Could you check a few things on this model? Use its own coordinates, in mm. A direction names the side the tool comes from. Round coordinates to 2 decimals unless told otherwise and drop trailing zeros. Order: outer loops, then holes, each group sorted by start corner. A loop starts at its lowest first (then second) coordinate and runs counter-clockwise, first axis right, second up. Notation, with made-up numbers: (84.25, 75.5) -> (90.25, 75.5) arc R23 cw to (90.25, 98.5) -> close; hole circle Ø4 at (-38.75, -6.5). An arc over 180 degrees is marked (long way). Put each result on its own line as item: value. Start each with the question number.
from build123d import *

# Parameters (mm, degrees)
BOSS_EXTRUDE1_DEPTH = 50
BOSS_EXTRUDE2_DEPTH = 30


with BuildPart() as part:
    # Sketch1 → Boss-Extrude1 (new body)
    with BuildSketch(Plane(origin=(0, 0, 0), x_dir=(1, 0, 0), z_dir=(0, 1, 0))):
        with BuildLine():
            Line((-1.5875, -2.749630657), (-1.5875, -22.749630657))
            Line((-1.5875, -22.749630657), (-5.5875, -22.749630657))
            Line((-5.5875, -22.749630657), (-5.5875, -4.501163044))
            ThreePointArc((-5.5875, -4.501163044), (0, 7.175), (5.5875, -4.501163044))
            Line((5.5875, -4.501163044), (5.5875, -22.749630657))
            Line((5.5875, -22.749630657), (1.5875, -22.749630657))
            Line((1.5875, -22.749630657), (1.5875, -2.749630657))
            ThreePointArc((1.5875, -2.749630657), (3.175, 0), (1.5875, 2.749630657))
            Line((1.5875, 2.749630657), (-1.5875, 2.749630657))
            ThreePointArc((-1.5875, 2.749630657), (-3.175, 0), (-1.5875, -2.749630657))
        make_face()
    extrude(amount=BOSS_EXTRUDE1_DEPTH)

    # Sketch5 → Boss-Extrude2 (add)
    with BuildSketch(Plane(origin=(0, 50, 0), x_dir=(1, 0, 0), z_dir=(0, 1, 0))):
        Polygon((-5.5875, -22.749630657), (-35.5875, -22.749630657), (-35.5875, -102.749630657), (-1.5875, -102.749630657), (-1.5875, -107.749630657), (-40.5875, -107.749630657), (-40.5875, -16.749630657), (-5.5875, -16.749630657), align=None)
    extrude(amount=-BOSS_EXTRUDE2_DEPTH)


solid = part.part
1. Thinking about a two-plate mould opening in X: for faces 5 (the face through (-1.588, 25, 13)), 6 (the face through (-40.588, 35, 63)), 7 (the face through (-36, 50, 50)), which applies, +X half, -X half, draft (parallel to the pull), parting line (faces both ways), or undercut?
2. If we section it at D-D, the plane z = 99: Please give me the cut outline in (x, y).
3. If we section it at B-B, the plane z = 12: Please give me the cut outline in (x, y).
4. For pin 1 Ø8 at (y, z) = (13, 12) entering from +X; pin 2 Ø10 at (x, y) = (-9.5, 18.5) entering from -Z; pin 3 Ø5.5 at (y, z) = (40.5, 106.5) entering from +X, each with a flat end and sliding along its axis, tell me the tip position at first contact or that it passes through.
5. I need wall thicknesses on L1, parallel to X at y = 38, z = 7; L2, parallel to Z at x = -13, y = 34; L3, parallel to Z at x = -4.5, y = 36. Which ranges of each line are inside material? Lowest first, please.
6. Which directions (+Z, -Z, +X, -X, +Y, -Y) give clear straight access to the entire face, cutting with the end or side of a thin tool? Please do faces 1 (the face through (0, 25, -2.75)), 2 (the face through (4, 25, 22.75)), 3 (the face through (-18, 36, 22.75)), 4 (the face through (3.175, 24.65, 0.047)).
7. If we section it at A-A, the plane x = -14.5: Please give me the cut outline in (y, z), then the cut area to 3 significant figures.
Results below:
1. face 5: undercut
1. face 6: -X half
1. face 7: draft
2. outline: (-40.59, 20) -> (-35.59, 20) -> (-35.59, 50) -> (-40.59, 50) -> close
3. outline: (-5.59, 0) -> (-1.59, 0) -> (-1.59, 50) -> (-5.59, 50) -> close; (1.59, 0) -> (5.59, 0) -> (5.59, 50) -> (1.59, 50) -> close
4. pin 1: x = 5.59
4. pin 2: z = -5.59
4. pin 3: x = -1.59
5. L1: -5.59 to -1.59, 1.59 to 5.59
5. L2: 16.75 to 22.75, 102.75 to 107.75
5. L3: -5.59 to 22.75, 102.75 to 107.75
6. face 1: +Z, +Y, -Y
6. face 2: +Z, +X, +Y, -Y
6. face 3: +X, +Y, -Y
6. face 4: +Y, -Y
7. outline: (20, 16.75) -> (50, 16.75) -> (50, 22.75) -> (20, 22.75) -> close; (20, 102.75) -> (50, 102.75) -> (50, 107.75) -> (20, 107.75) -> close
7. area: 330 mm2
